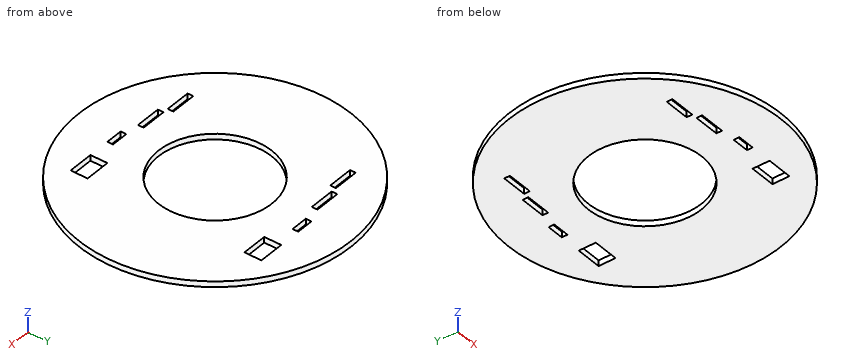
```python
from build123d import *

# Parameters (mm, degrees)
SKETCH1_R           = 76.2
SKETCH1_R_2         = 31.75
BOSS_EXTRUDE1_DEPTH = 3.175
CAVITY1_START       = -53.511255689
CAVITY1_OUTLINE_W   = 14.2875
CAVITY1_OUTLINE_H   = 3.175
CAVITY1_DEPTH       = 9.525
CAVITY1_START_2     = 43.986255689
CAVITY1_2_OUTLINE_W = 14.2875
CAVITY1_2_OUTLINE_H = 3.175
CAVITY1_2_DEPTH     = 9.525
CAVITY1_START_3     = -50.336255689
CAVITY1_3_OUTLINE_W = 14.2875
CAVITY1_3_OUTLINE_H = 3.175
CAVITY1_3_DEPTH     = 3.175
CAVITY1_START_4     = -47.161255689
CAVITY1_4_OUTLINE_W = 14.2875
CAVITY1_4_OUTLINE_H = 3.175
CAVITY1_4_DEPTH     = 3.175
CAVITY1_5_OUTLINE_W = 14.2875
CAVITY1_5_OUTLINE_H = 3.175
CAVITY1_5_DEPTH     = 3.175
CAVITY1_START_5     = 47.161255689
CAVITY1_6_OUTLINE_W = 14.2875
CAVITY1_6_OUTLINE_H = 3.175
CAVITY1_6_DEPTH     = 3.175
CAVITY1_7_OUTLINE_W = 9.525
CAVITY1_7_OUTLINE_H = 3.175
CAVITY1_7_DEPTH     = 3.175
CAVITY1_START_6     = 50.336255689
CAVITY1_8_OUTLINE_W = 9.525
CAVITY1_8_OUTLINE_H = 3.175
CAVITY1_8_DEPTH     = 3.175


# Read off the part's stored shape, not the designer's step: Cavity1
with BuildPart() as part:
    # Sketch1 → Boss-Extrude1 (new body)
    with BuildSketch(Plane.XY):
        Circle(SKETCH1_R)
        Circle(SKETCH1_R_2, mode=Mode.SUBTRACT)
    extrude(amount=BOSS_EXTRUDE1_DEPTH)

    # Cavity1 outline → Cavity1 (cut)
    with BuildSketch(Plane(origin=(0, 0, 0), x_dir=(0.9999649697426024, 0.008370142631770718, 0), z_dir=(0.008370142631770716, -0.9999649697426025, 0)).offset(CAVITY1_START)):
        with Locations((28.254299641, 1.5875)):
            Rectangle(CAVITY1_OUTLINE_W, CAVITY1_OUTLINE_H)
    extrude(amount=CAVITY1_DEPTH, mode=Mode.SUBTRACT)

    # Cavity1 2 outline → Cavity1 2 (cut)
    with BuildSketch(Plane(origin=(0, 0, 0), x_dir=(0.9999649697426024, 0.008370142631770718, 0), z_dir=(0.008370142631770716, -0.9999649697426025, 0)).offset(CAVITY1_START_2)):
        with Locations((28.254299641, 1.5875)):
            Rectangle(CAVITY1_2_OUTLINE_W, CAVITY1_2_OUTLINE_H)
    extrude(amount=CAVITY1_2_DEPTH, mode=Mode.SUBTRACT)

    # Cavity1 3 outline → Cavity1 3 (cut)
    with BuildSketch(Plane(origin=(0, 0, 0), x_dir=(0.9999649697426024, 0.008370142631770718, 0), z_dir=(0.008370142631770716, -0.9999649697426025, 0)).offset(CAVITY1_START_3)):
        with Locations((-16.280608677, 1.5875)):
            Rectangle(CAVITY1_3_OUTLINE_W, CAVITY1_3_OUTLINE_H)
    extrude(amount=CAVITY1_3_DEPTH, mode=Mode.SUBTRACT)

    # Cavity1 4 outline → Cavity1 4 (cut)
    with BuildSketch(Plane(origin=(0, 0, 0), x_dir=(0.9999649697426024, 0.008370142631770718, 0), z_dir=(0.008370142631770716, -0.9999649697426025, 0)).offset(CAVITY1_START_4)):
        with Locations((-33.658200359, 1.5875)):
            Rectangle(CAVITY1_4_OUTLINE_W, CAVITY1_4_OUTLINE_H)
    extrude(amount=CAVITY1_4_DEPTH, mode=Mode.SUBTRACT)

    # Cavity1 5 outline → Cavity1 5 (cut)
    with BuildSketch(Plane(origin=(0, 0, 0), x_dir=(0.9999649697426024, 0.008370142631770718, 0), z_dir=(0.008370142631770716, -0.9999649697426025, 0)).offset(CAVITY1_START_2)):
        with Locations((-33.658200359, 1.5875)):
            Rectangle(CAVITY1_5_OUTLINE_W, CAVITY1_5_OUTLINE_H)
    extrude(amount=CAVITY1_5_DEPTH, mode=Mode.SUBTRACT)

    # Cavity1 6 outline → Cavity1 6 (cut)
    with BuildSketch(Plane(origin=(0, 0, 0), x_dir=(0.9999649697426024, 0.008370142631770718, 0), z_dir=(0.008370142631770716, -0.9999649697426025, 0)).offset(CAVITY1_START_5)):
        with Locations((-16.280608677, 1.5875)):
            Rectangle(CAVITY1_6_OUTLINE_W, CAVITY1_6_OUTLINE_H)
    extrude(amount=CAVITY1_6_DEPTH, mode=Mode.SUBTRACT)

    # Cavity1 7 outline → Cavity1 7 (cut)
    with BuildSketch(Plane(origin=(0, 0, 0), x_dir=(0.9999649697426024, 0.008370142631770718, 0), z_dir=(0.008370142631770716, -0.9999649697426025, 0)).offset(CAVITY1_START)):
        with Locations((4.078332174, 1.5875)):
            Rectangle(CAVITY1_7_OUTLINE_W, CAVITY1_7_OUTLINE_H)
    extrude(amount=CAVITY1_7_DEPTH, mode=Mode.SUBTRACT)

    # Cavity1 8 outline → Cavity1 8 (cut)
    with BuildSketch(Plane(origin=(0, 0, 0), x_dir=(0.9999649697426024, 0.008370142631770718, 0), z_dir=(0.008370142631770716, -0.9999649697426025, 0)).offset(CAVITY1_START_6)):
        with Locations((4.078332174, 1.5875)):
            Rectangle(CAVITY1_8_OUTLINE_W, CAVITY1_8_OUTLINE_H)
    extrude(amount=CAVITY1_8_DEPTH, mode=Mode.SUBTRACT)


solid = part.part
```
For this review, take the finished solid that the model builds, in its own axes (mm). Give positions to 0.01 mm unless a question says otherwise; leave off trailing zeros. Loops run counter-clockwise (first coordinate to the right, second up) from the corner with the lowest first, then second, coordinate; pieces in that order, holes last. Notation, with made-up numbers: M 46.25,65 L 101.25,65 A6 cw 101.25,75 Z; hole C 69.25,35.5 d4. An arc over 180 degrees is marked long. One line per item, written item: value. Start each with the question number.
Q1. Add section B-B (z = 0.5). Count the separate pieces of the cut face and the enclosed holes in it, and give its area (3 significant figures).
Q2. Add section D-D (y = -56). Give the boundary of the cut face in (x, z) (3 decimals), and give its area (3 significant figures).
Q3. Add section A-A (y = 0). Give the boundary of the cut face in (x, z) (3 decimals).
Q4. Clearance check with flat-ended pins moving along their axes: pin 1 Ø1.5 at (x, z) = (-27, 1.5) entering from -Y; pin 2 Ø1.5 at (y, z) = (-38.5, 1) entering from +X. State where each tip first meets the part, or that it passes through.
Q5. For L1, parallel to Y at x = -0.5, z = 1.95; L2, parallel to Y at x = 0, z = 1.05; L3, parallel to X at y = -47, z = 2.4, list the stretches that pass through material, from the lowest coordinate up.
Q6. Add section C-C (x = -53). Give the boundary of the cut face in (y, z) (3 decimals), and give its area (3 significant figures).
Reply:
1. separate pieces: 1
1. enclosed holes: 9
1. area: 14,600 mm²
2. outline: M -51.676,0 L 51.676,0 L 51.676,3.175 L -51.676,3.175 Z
2. area: 328 mm²
3. outline: M -76.2,0 L -31.75,0 L -31.75,3.175 L -76.2,3.175 Z; M 31.75,0 L 76.2,0 L 76.2,3.175 L 31.75,3.175 Z
4. pin 1: y = -71.54
4. pin 2: x = 66.19
5. L1: -76.2 to -31.75, 31.75 to 50.33, 53.51 to 76.2
5. L2: -76.2 to -53.51, -50.34 to -31.75, 31.75 to 50.34, 53.51 to 76.2
5. L3: -59.98 to -40.41, -26.12 to 21.5, 35.79 to 59.98
6. outline: M -54.749,0 L 54.749,0 L 54.749,3.175 L -54.749,3.175 Z
6. area: 348 mm²
